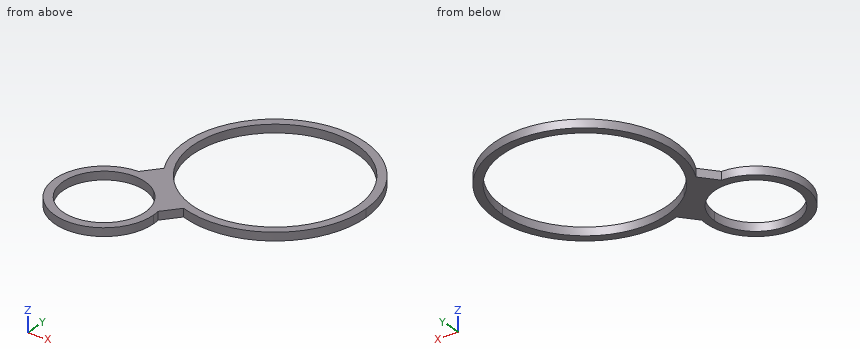
from build123d import *

# Parameters (mm, degrees)
F1_DEPTH = 3


with BuildPart() as f1:
    # F0 (on Top) → F1 (new body)
    with BuildSketch(Plane.XY):
        with BuildLine():
            ThreePointArc((-15.755804, -37.070002), (-17.804677, -30.868516), (-21.931504, -25.806342))
            ThreePointArc((-21.931504, -25.806342), (-27.592968, -22.549942), (-34.043707, -21.528038))
            ThreePointArc((-34.043707, -21.528038), (-46.153741, -52.410308), (-15.587977, -39.522268))
            ThreePointArc((-15.587977, -39.522268), (-15.629983, -38.293267), (-15.755804, -37.070002))
        make_face()
        with BuildLine():
            ThreePointArc((-18.587977, -39.522268), (-47.202416, -45.818858), (-23.87425, -28.092329))
            ThreePointArc((-23.87425, -28.092329), (-19.973538, -33.225678), (-18.587977, -39.522268))
        make_face(mode=Mode.SUBTRACT)
        with BuildLine():
            ThreePointArc((-29.051168, -15.653423), (-25.653561, -20.758006), (-21.3702, -25.145866))
            ThreePointArc((-21.3702, -25.145866), (-16.348978, -28.665501), (-10.763265, -31.195386))
            ThreePointArc((-10.763265, -31.195386), (19.154794, -26.871805), (33, 0))
            ThreePointArc((33, 0), (-8.07191, 31.997567), (-29.051168, -15.653423))
        make_face()
        with BuildLine():
            ThreePointArc((-19.427454, -22.859878), (-12.59318, 27.228878), (30, 0))
            ThreePointArc((30, 0), (12.59318, -27.228878), (-19.427454, -22.859878))
        make_face(mode=Mode.SUBTRACT)
        with BuildLine():
            ThreePointArc((-10.763265, -31.195386), (-16.348978, -28.665501), (-21.3702, -25.145866))
            Line((-21.3702, -25.145866), (-21.931504, -25.806342))
            ThreePointArc((-21.931504, -25.806342), (-17.804677, -30.868516), (-15.755804, -37.070002))
            Line((-15.755804, -37.070002), (-10.763265, -31.195386))
        make_face()
        with BuildLine():
            Line((-21.931504, -25.806342), (-21.3702, -25.145866))
            ThreePointArc((-21.3702, -25.145866), (-25.653561, -20.758006), (-29.051168, -15.653423))
            Line((-29.051168, -15.653423), (-34.043707, -21.528038))
            ThreePointArc((-34.043707, -21.528038), (-27.592968, -22.549942), (-21.931504, -25.806342))
        make_face()
    extrude(amount=F1_DEPTH)


solid = f1.part
Design review of the part built by this model. Coordinates are the model's own, in mm. Give positions to 0.01 mm unless a question says otherwise; leave off trailing zeros. Loops run counter-clockwise (first coordinate to the right, second up) from the corner with the lowest first, then second, coordinate; pieces in that order, holes last. Notation, with made-up numbers: (8, 8) -> (65, 8) arc R19 cw to (65, 31) -> close; hole circle Ø8 at (-14, 47.5). An arc over 180 degrees is marked (long way). One line per question, with ' | ' between items. Start each with the question number.
(1) We need section D-D (x = -21). State the section outline as (y, z) points.
(2) Insertion check: P1, Ø1, axis at x = 9.5, z = 1, coming from the +Y side; P2, Ø1, axis at x = 20, z = 1, coming from the +Y side. Each pin has a flat end and moves straight along its axis. Give the tip position at first contact, or say it passes through.
(3) We need section A-A (x = 0). State the section outline as (y, z) points, and give its area (3 significant figures).
(4) We need section B-B (z = 0.6). State the section outline as (x, y) points.
(5) We need section C-C (y = -49). State the section outline as (x, z) points, and give its area (3 significant figures).
(6) For line 1 (Y direction, x = 0, z = 1.45); line 2 (X direction, y = 9, z = 1.2); line 3 (X direction, y = 14.5, z = 0.3), list the stretches that pass through material, from the lowest coordinate up.
The answers:
1) outline: (-52.39, 0) -> (-47.68, 0) -> (-47.68, 3) -> (-52.39, 3) -> close; (-31.36, 0) -> (-21.42, 0) -> (-21.42, 3) -> (-31.36, 3) -> close; (21.42, 0) -> (25.46, 0) -> (25.46, 3) -> (21.42, 3) -> close
2) P1: stops at y = 31.75 | P2: stops at y = 26.62
3) outline: (-33, 0) -> (-30, 0) -> (-30, 3) -> (-33, 3) -> close; (30, 0) -> (33, 0) -> (33, 3) -> (30, 3) -> close | area: 18.0 mm^2
4) outline: (-34.04, -21.53) arc R18 ccw (long way) to (-15.59, -39.52) arc R18 ccw to (-15.76, -37.07) -> (-10.76, -31.2) arc R33 ccw to (33, 0) arc R33 ccw (long way) to (-29.05, -15.65) -> close; hole circle Ø60 at (0, 0); hole (-23.87, -28.09) arc R15 ccw (long way) to (-18.59, -39.52) arc R15 ccw to start
5) outline: (-48.89, 0) -> (-45.21, 0) -> (-45.21, 3) -> (-48.89, 3) -> close; (-21.96, 0) -> (-18.29, 0) -> (-18.29, 3) -> (-21.96, 3) -> close | area: 22.1 mm^2
6) line 1: y = -33 to -30, 30 to 33 | line 2: x = -31.75 to -28.62, 28.62 to 31.75 | line 3: x = -29.64 to -26.26, 26.26 to 29.64
